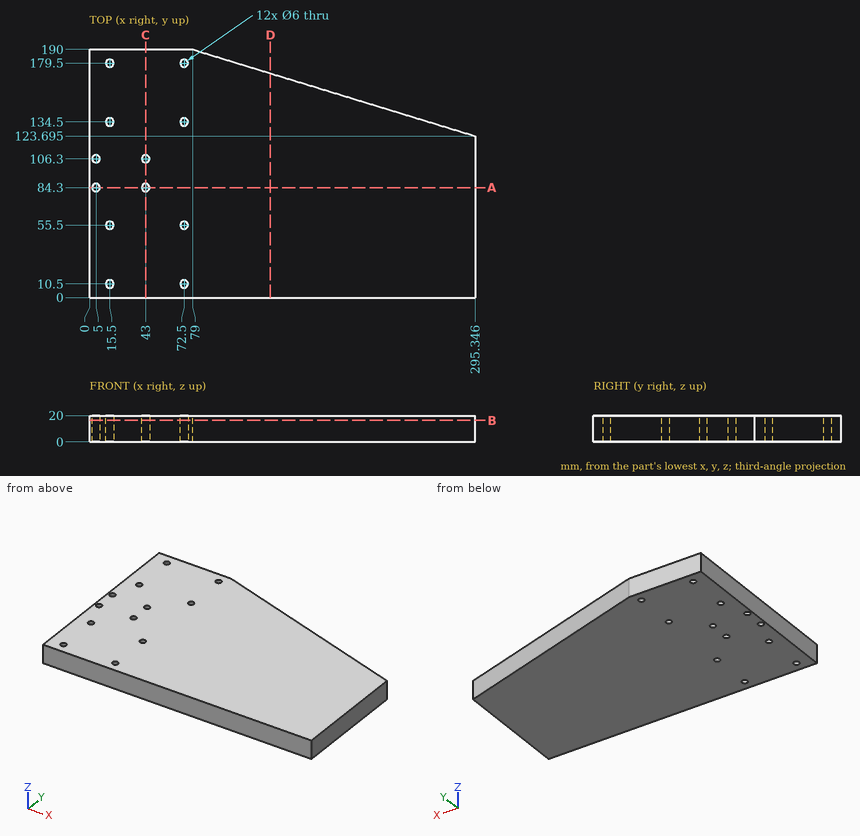
Study the drawing (mm; zero at the part's minimum x, y, z) and answer. Coordinates: 2 decimals unless noted, no trailing zeros. Loops run counter-clockwise (first coordinate to the right, second up) from the corner with the lowest first, then second, coordinate; pieces in that order, holes last. Notation, with made-up numbers: M -30.75,-16 L 2.25,-16 A18 cw 2.25,17 Z; hole C 38,-33 d10. An arc over 180 degrees is marked long. Answer in a Markdown table with one row per item. Add a question column.
1. Find section A-A, the plane y = 84.3. Write down the section's boundary in (x, z), then the cut area to 3 significant figures.
2. Find section B-B, the plane z = 16.5. State how many separate pieces and enclosed holes the cut face has, then the cut area to 3 significant figures.
3. A flat-ended cylindrical pin translates along its axis: P1, Ø10, axis at x = 176, z = 9, coming from the +Y side. Find the tip coordinate at first contact, or state that the pin passes through.
4. Find section D-D, the plane x = 138.5. Write down the section's boundary in (y, z) (1 decimal).
5. Find section C-C, the plane x = 43. Write down the section's boundary in (y, z), then the cut area to 3 significant figures.
6. Consider L1, parallel to Y at x = 5, z = 12; L2, parallel to Y at x = 15.5, z = 15; L3, parallel to X at y = 58, z = 5.25 (1 decimal). Determine where each line is inside the solid, lowest interval first.
Reported:
| question | item | result |
|---|---|---|
| 1 | outline | M 0,0 L 2,0 L 2,20 L 0,20 Z; M 8,0 L 40,0 L 40,20 L 8,20 Z; M 46,0 L 295.35,0 L 295.35,20 L 46,20 Z |
| 1 | area | 5,670 mm^2 |
| 2 | separate pieces | 1 |
| 2 | enclosed holes | 12 |
| 2 | area | 48,600 mm^2 |
| 3 | P1 | stops at y = 161.8 |
| 4 | outline | M 0,0 L 171.8,0 L 171.8,20 L 0,20 Z |
| 5 | outline | M 0,0 L 81.3,0 L 81.3,20 L 0,20 Z; M 87.3,0 L 103.3,0 L 103.3,20 L 87.3,20 Z; M 109.3,0 L 190,0 L 190,20 L 109.3,20 Z |
| 5 | area | 3,560 mm^2 |
| 6 | L1 | y = 0 to 81.3, 87.3 to 103.3, 109.3 to 190 |
| 6 | L2 | y = 0 to 7.5, 13.5 to 52.5, 58.5 to 131.5, 137.5 to 176.5, 182.5 to 190 |
| 6 | L3 | x = 0 to 13.8, 17.2 to 70.8, 74.2 to 295.3 |
